from build123d import *

# Parameters (mm, degrees)
F0_W     = 420
F0_H     = 210
F1_DEPTH = 150
F3_DEPTH = 420.001
F4_R     = 4
F5_DEPTH = 15
F7_DEPTH = 150


with BuildPart() as f1:
    # F0 (on Top) → F1 (new body)
    with BuildSketch(Plane.XY):
        with Locations((210, -105)):
            Rectangle(F0_W, F0_H)
    extrude(amount=F1_DEPTH)

    # F2 (on face) → F3 (cut, through all)
    with BuildSketch(Plane.YZ.offset(420)):
        Polygon((-210, 150), (-210, 75), (-123.2505664229, 150), align=None)
    extrude(amount=-F3_DEPTH, mode=Mode.SUBTRACT)

    # F4 (on face) → F5 (cut)
    with BuildSketch(Plane(origin=(0, -126.9320637805, 146.8171284764), x_dir=(1, 0, 0), z_dir=(0, -0.6540195362, 0.7564776575))):
        with Locations((45.6720627844, -23.2154857367)):
            Circle(F4_R)
        with Locations((66.2421623061, -23.3697257936)):
            Circle(F4_R)
        with Locations((67.1772722169, -40.1790748625)):
            Circle(F4_R)
        with Locations((45.5067284684, -40.0792160809)):
            Circle(F4_R)
        with BuildLine():
            Line((123.8630712032, -20.2180277556), (96.6224558651, -20.2180277556))
            ThreePointArc((96.6224558651, -20.2180277556), (93.0059849426, -21.7160190597), (91.5079936385, -25.3324899822))
            Line((91.5079936385, -25.3324899822), (91.5079936385, -90.4371738434))
            ThreePointArc((91.5079936385, -90.4371738434), (92.9668696589, -93.9592121177), (96.4889079332, -95.4180881381))
            Line((96.4889079332, -95.4180881381), (123.4852224588, -95.4180881381))
            ThreePointArc((123.4852224588, -95.4180881381), (127.2878428404, -93.8429912035), (128.862939775, -90.040370822))
            Line((128.862939775, -90.040370822), (128.862939775, -25.2178963274))
            ThreePointArc((128.862939775, -25.2178963274), (127.3985121754, -21.6824553552), (123.8630712032, -20.2180277556))
        make_face()
    extrude(amount=-F5_DEPTH, mode=Mode.SUBTRACT)

    # F6 (on face) → F7 (cut)
    with BuildSketch(Plane.YZ.offset(420)):
        Polygon((-206.3629985005, 78.1444022308), (-210, 75), (0, 75), (0, 150), (-123.2505664229, 150), align=None)
    extrude(amount=-F7_DEPTH, mode=Mode.SUBTRACT)


solid = f1.part
Source: CAD feature listing. Evaluate the final solid. Frame: model axes, mm. A direction names the side the tool comes from. Coordinates: 2 decimals unless noted, no trailing zeros. Write each loop counter-clockwise with the first axis right and the second up, starting at its lowest first coordinate (ties: lowest second). Pieces come first, ordered by that corner, then holes. Notation, with made-up numbers: M 21,72.25 L 31,72.25 A28 cw 31,93.25 Z; hole C 54.25,82 d9. An arc over 180 degrees is marked long. Use a Markdown table: item, result.
1) Section A-A, the plane y = -44. Output: boundary loops of the cut face in (x, z).
Conclusion:
| item | result |
|---|---|
| outline | M 0,0 L 420,0 L 420,75 L 270,75 L 270,150 L 0,150 Z |
2) Mould query, pull axis Y, two halves, no side actions, for faces 5 (the cylindrical face through (92.928, -193.144, 79.797)), 6 (the flat face through (207, -104, 0)), 7 (the flat face through (207, -210, 37)). Classes: pulls with the +Y half, pulls with the -Y half, needs draft (parallel to the pull), parting line crosses it, or undercut.
Conclusion:
| item | result |
|---|---|
| face 5 | undercut |
| face 6 | needs draft |
| face 7 | pulls with the -Y half |
3) First-contact query: pin 1 Ø6 at (x, y) = (171, -29.5) entering from -Z; pin 2 Ø10 at (x, y) = (104, -179) entering from +Z; pin 3 Ø1.5 at (x, y) = (87, -141) entering from +Z. Flat tips, straight axial feed; report the tip coordinate or a pass-through.
Conclusion:
| item | result |
|---|---|
| pin 1 | stops at z = 0 |
| pin 2 | stops at z = 86.3 |
| pin 3 | stops at z = 135.3 |
4) Section C-C, the plane x = 283.5. Output: boundary loops of the cut face in (y, z), then the cut area to 4 significant figures.
Conclusion:
| item | result |
|---|---|
| outline | M -210,0 L 0,0 L 0,75 L -210,75 Z |
| area | 15,750 mm^2 |
5) Reachability of faces 1 (the cylindrical face through (127.246, -193.117, 79.821)), 2 (the flat face through (0, -106, 74)), 3 (the flat face through (346, -106, 75)), 4 (the cylindrical face through (93.05, -138.49, 127.05)) from +Z, -Z, +X, -X, +Y, -Y: full face, straight path, thin tool, end or side. Return the list, or none.
Conclusion:
| item | result |
|---|---|
| face 1 | +Z |
| face 2 | +Z, -Z, -X, +Y, -Y |
| face 3 | +Z, +X, +Y, -Y |
| face 4 | -Y |
6) Ray query, L1, parallel to X at y = -79, z = 140; L2, parallel to Z at x = 315, y = -61.5; L3, parallel to Y at x = 28, z = 134. Return the intervals inside material, ascending.
Conclusion:
| item | result |
|---|---|
| L1 | x = 0 to 270 |
| L2 | z = 0 to 75 |
| L3 | y = -141.76 to 0 |
7) Section B-B, the plane x = 237. Output: boundary loops of the cut face in (y, z).
Conclusion:
| item | result |
|---|---|
| outline | M -210,0 L 0,0 L 0,150 L -123.25,150 L -210,75 Z |
